Verification items for the finished model (mm, model axes). Give positions to 0.01 mm unless a question says otherwise; leave off trailing zeros. Loops run counter-clockwise (first coordinate to the right, second up) from the corner with the lowest first, then second, coordinate; pieces in that order, holes last. Notation, with made-up numbers: (-27.5, 7) - (-14.5, 7) arc R28 cw to (-14.5, 27) - close; hole circle Ø9 at (63, 26). An arc over 180 degrees is marked (long way). One line per item, written item: value. Start each with the question number.
1. Scan lines: L1, parallel to Z at x = 23.5, y = 1.35; L2, parallel to X at y = 1.3, z = 8; L3, parallel to Z at x = -1.5, y = 0.7. Record each from-to range of solid material in increasing order. Write a range as [from, to].
2. Mould release check, pull along X, two halves, no side actions. Record for faces 1 (the cylindrical face through (-60.47, 1.252, 46.367)), 2 (the cylindrical face through (34.1, 1.3, 50.4)), 3 (the flat face through (-1, 2.54, -1)): pulls with the +X half, pulls with the -X half, needs draft (parallel to the pull), parting line crosses it, or undercut.
3. Sectioned sample at A-A (x = 56.5). Record the cut outline in (y, z).
4. Gauge pin test, flat ends, axial feed: pin 1 (5.5 mm diameter, centred on x = -9.31, z = -23.63, fed in from -Y); pin 2 (1.5 mm diameter, centred on x = -51, y = 2, fed in from -Z). Record the tip position at first contact, or that the pin passes through.
5. Sectioned sample at B-B (y = 1.5). Count the separate pieces of the cut face and the enclosed holes in it, plus the area to 3 significant figures.
6. Sectioned sample at C-C (x = -23). Record the cut outline in (y, z), plus the area to 3 significant figures.
7. Sectioned sample at D-D (z = -34.5). Record the cut outline in (x, y), plus the area to 3 significant figures.
from build123d import *

# Parameters (mm, degrees)
SKETCH1_R           = 76.2
BOSS_EXTRUDE1_DEPTH = 2.54
SKETCH2_R           = 3.175
CUT_EXTRUDE1_DEPTH  = 2.54
SKETCH4_R           = 3.175
CUT_EXTRUDE3_DEPTH  = 3.54


with BuildPart() as part:
    # Sketch1 → Boss-Extrude1 (new body)
    with BuildSketch(Plane(origin=(0, 0, 0), x_dir=(1, 0, 0), z_dir=(0, 1, 0))):
        Circle(SKETCH1_R)
    extrude(amount=BOSS_EXTRUDE1_DEPTH)

    # Sketch2 → Cut-Extrude1 (cut)
    with BuildSketch(Plane.XZ):
        with Locations((-67.814061825, 8.585318756)):
            Circle(SKETCH2_R)
        with Locations((-41.97979671, -50.809492852)):
            Circle(SKETCH2_R)
        with Locations((57.01155597, -7.752384327)):
            Circle(SKETCH2_R)
        with Locations((31.177290855, 51.642427281)):
            Circle(SKETCH2_R)
    extrude(amount=-CUT_EXTRUDE1_DEPTH, mode=Mode.SUBTRACT)

    # Sketch4 → Cut-Extrude3 (cut, through all)
    with BuildSketch(Plane(origin=(0, 2.54, 0), x_dir=(1, 0, 0), z_dir=(0, 1, 0))):
        with Locations((-9.306231375, 23.633748277)):
            Circle(SKETCH4_R)
        with Locations((23.633748277, 9.306231375)):
            Circle(SKETCH4_R)
        with Locations((9.306231375, -23.633748277)):
            Circle(SKETCH4_R)
        with Locations((-23.633748277, -9.306231375)):
            Circle(SKETCH4_R)
    extrude(amount=-CUT_EXTRUDE3_DEPTH, mode=Mode.SUBTRACT)


solid = part.part
Results are:
1. L1: z = [-72.49, -12.48], [-6.13, 72.49]
1. L2: x = [-75.78, -70.93], [-64.69, -26.53], [-20.74, 75.78]
1. L3: z = [-76.19, 76.19]
2. face 1: parting line crosses it
2. face 2: undercut
2. face 3: needs draft
3. outline: (0, -51.13) - (2.54, -51.13) - (2.54, -10.89) - (0, -10.89) - close; (0, -4.62) - (2.54, -4.62) - (2.54, 51.13) - (0, 51.13) - close
4. pin 1: passes through
4. pin 2: stops at z = -57.28
5. separate pieces: 1
5. enclosed holes: 8
5. area: 18,000 mm^2
6. outline: (0, -72.65) - (2.54, -72.65) - (2.54, 6.2) - (0, 6.2) - close; (0, 12.42) - (2.54, 12.42) - (2.54, 72.65) - (0, 72.65) - close
6. area: 353 mm^2
7. outline: (-67.94, 0) - (67.94, 0) - (67.94, 2.54) - (-67.94, 2.54) - close
7. area: 345 mm^2
